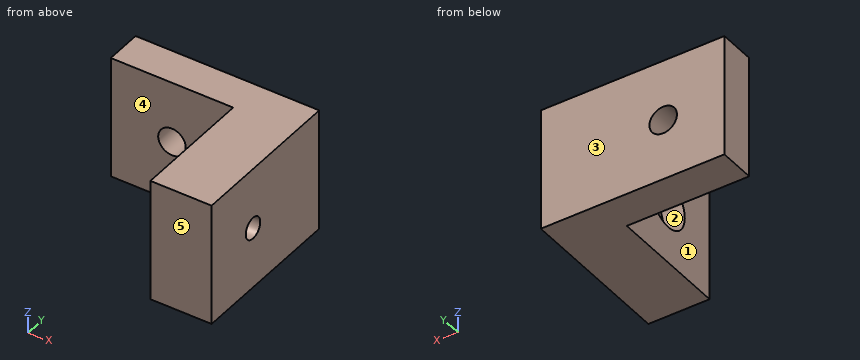
from build123d import *

# Parameters (mm, degrees)
PAD_DEPTH       = 20
SKETCH001_R     = 2.25
POCKET_DEPTH    = 6.001
SKETCH002_R     = 1.75
POCKET001_DEPTH = 10.001
SKETCH003_R     = 4
POCKET002_DEPTH = 3.5


with BuildPart() as part:
    # Sketch → Pad (new body)
    with BuildSketch(Plane.XY):
        Polygon((0, 0), (0, -20), (10, -20), (10, 6), (-20, 6), (-20, 0), align=None)
    extrude(amount=PAD_DEPTH)

    # Sketch001 → Pocket (cut, through all)
    with BuildSketch(Plane.XZ):
        with Locations((-10, 10)):
            Circle(SKETCH001_R)
    extrude(amount=-POCKET_DEPTH, mode=Mode.SUBTRACT)

    # Sketch002 → Pocket001 (cut, through all)
    with BuildSketch(Plane(origin=(0, 0, 0), x_dir=(0, -1, 0), z_dir=(-1, 0, 0))):
        with Locations((10, 10)):
            Circle(SKETCH002_R)
    extrude(amount=-POCKET001_DEPTH, mode=Mode.SUBTRACT)

    # Sketch003 → Pocket002 (cut)
    with BuildSketch(Plane(origin=(0, 0, 0), x_dir=(0, -1, 0), z_dir=(-1, 0, 0))):
        with Locations((10, 10)):
            Circle(SKETCH003_R)
    extrude(amount=-POCKET002_DEPTH, mode=Mode.SUBTRACT)


solid = part.part
Can you work these out from the model? Positions are in its coordinate system, mm. Face numbers are marked on the shaded views. A direction names the side the tool comes from. Coordinates: 2 decimals unless noted, no trailing zeros. Write each loop counter-clockwise with the first axis right and the second up, starting at its lowest first coordinate (ties: lowest second). Pieces come first, ordered by that corner, then holes. Notation, with made-up numbers: (66, 48.5) -> (124, 48.5) arc R37 ccw to (124, 87.5) -> close; hole circle Ø11 at (53.5, 19). An arc over 180 degrees is marked (long way). Write each question's results on one line, items separated by ' | '. Start each with the question number.
Item 1: Please list where these lines run through material, in increasing order: probe 1 along Z at (x, y) = (6.5, -10); probe 2 along Z at (x, y) = (-10, 4.35); probe 3 along Y at (x, z) = (-12, 4.25).
Item 2: Thinking about a two-plate mould opening in Y: for the marked faces 1, 2 and 3, which applies, released by +Y, released by -Y, zero draft, split by the parting line, or undercut?
Item 3: I'm going to push flat-ended pins straight in: P1, Ø6.5, axis at y = -10, z = 10, coming from the +X side; P2, Ø4, axis at y = -11, z = 8.5, coming from the -X side; P3, Ø3, axis at y = -7, z = 17.5, coming from the -X side; P4, Ø10, axis at x = -9.5, z = 10.5, coming from the -Y side. Where does each tip first touch, or does it pass through?
Item 4: If we section it at A-A, the plane z = 10: Write out the boundary of the cut face in (x, y).
Item 5: On a 3-axis mill with a long thin cutter (end or side, diameter ignored), from which of +Z, -Z, +X, -X, +Y, -Y can I reach the whole of each face in a straight line? I mean the marked faces 4 and 5. Say none if no direction works.
Item 6: If we section it at B-B, the plane x = -10: Write out the boundary of the cut face in (y, z), and give its area (3 significant figures).
Item 7: If we section it at D-D, the plane y = 3.75: Write out the boundary of the cut face in (x, z), and give its area (3 significant figures).
Item 8: If we section it at C-C, the plane y = -10: Write out the boundary of the cut face in (x, z).
Answer block:
1) probe 1: 0 to 8.25, 11.75 to 20 | probe 2: 0 to 7.75, 12.25 to 20 | probe 3: 0 to 6
2) face 1: zero draft | face 2: undercut | face 3: released by +Y
3) P1: x = 10 | P2: x = 3.5 | P3: x = 0 | P4: y = 0
4) outline: (-20, 0) -> (-12.25, 0) -> (-12.25, 6) -> (-20, 6) -> close; (-7.75, 0) -> (0, 0) -> (0, -6) -> (3.5, -6) -> (3.5, -8.25) -> (10, -8.25) -> (10, 6) -> (-7.75, 6) -> close; (0, -20) -> (10, -20) -> (10, -11.75) -> (3.5, -11.75) -> (3.5, -14) -> (0, -14) -> close
5) face 4: +Z, -Z, -X, -Y | face 5: +Z, -Z, +X, -X, -Y
6) outline: (0, 0) -> (6, 0) -> (6, 7.75) -> (0, 7.75) -> close; (0, 12.25) -> (6, 12.25) -> (6, 20) -> (0, 20) -> close | area: 93.0 mm²
7) outline: (-20, 0) -> (10, 0) -> (10, 20) -> (-20, 20) -> close; hole circle Ø4.5 at (-10, 10) | area: 584 mm²
8) outline: (0, 0) -> (10, 0) -> (10, 8.25) -> (3.5, 8.25) -> (3.5, 6) -> (0, 6) -> close; (0, 14) -> (3.5, 14) -> (3.5, 11.75) -> (10, 11.75) -> (10, 20) -> (0, 20) -> close
